Geometry check sheet. Reference: the model listing, model coordinates, mm. Give positions to 0.01 mm unless a question says otherwise; leave off trailing zeros. Order: outer loops, then holes, each group sorted by start corner. A loop starts at its lowest first (then second) coordinate and runs counter-clockwise, first axis right, second up. Notation, with made-up numbers: M 6.5,17 L 16.5,17 A26 ccw 16.5,42 Z; hole C -5,10 d2. An arc over 180 degrees is marked long. Answer as CSV lines item,"result". Start each with the question number.
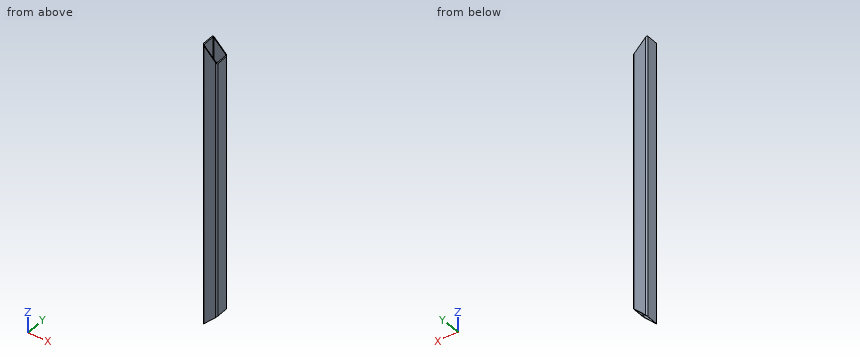
Autodesk Inventor part; units mm, degrees
ref_plane "Piano iniziale" through (0, 0, 0) normal (0, 0, 1) x (1, 0, 0)
ref_plane "Piano finale" through (0, 0, 800) normal (0, 0, 1) x (1, 0, 0)
ref_plane "YZ Plane" through (0, 0, 0) normal (1, 0, 0) x (0, 1, 0)
ref_plane "Piano iniziale" through (0, 0, 0) normal (0, 0, 1) x (1, 0, 0)
ref_plane "Piano finale" through (0, 0, 800) normal (0, 0, 1) x (1, 0, 0)
sketch "Schizzo" plane through (0, 0, 0) normal (0, 0, 1) x (1, 0, 0)
  line L0 (-20, -16) -> (-20, 16)
  line L1 (-16, 20) -> (16, 20)
  line L2 (20, 16) -> (20, -16)
  line L3 (16, -20) -> (-16, -20)
  arc A0 (-20, -16) -> (-16, -20) centre (-16, -16) ccw
  arc A1 (20, 16) -> (16, 20) centre (16, 16) ccw
  arc A2 (-16, 20) -> (-20, 16) centre (-16, 16) ccw
  arc A3 (16, -20) -> (20, -16) centre (16, -16) ccw
  arc A4 (-16, 18) -> (-18, 16) centre (-16, 16) ccw
  line L4 (-16, 18) -> (16, 18)
  arc A5 (18, 16) -> (16, 18) centre (16, 16) ccw
  line L5 (18, 16) -> (18, -16)
  arc A6 (16, -18) -> (18, -16) centre (16, -16) ccw
  line L6 (16, -18) -> (-16, -18)
  arc A7 (-18, -16) -> (-16, -18) centre (-16, -16) ccw
  line L7 (-18, -16) -> (-18, 16)
  line L8 (0, 29.1598) -> (0, -29.1598) construction
  line L9 (-29.1598, 0) -> (29.1598, 0) construction
  dimension "d7" = 4
  dimension "d9" = 40
  dimension "d11" = 40
  dimension "d12" = 2
  dimension "d15" = 20
  dimension "d16" = 20
extrude "Corpo" add sketch "Schizzo" along normal up to surface (800 mm away) from surface at 0
sketch "Sketch3" plane through (0, 0, 0) normal (0, 0, 1) x (1, 0, 0)
  line L0 (0, 0) -> (10, 0)
ref_plane "Work Plane3" through (0, 0, 0) normal (0, -1, 0) x (1, 0, 0)
sketch "Sketch4" plane through (0, 0, 0) normal (0, -1, 0) x (1, 0, 0)
  line L0 (-2, 0) -> (12, 0)
  line L1 (-2, 800) -> (12, 800)
  dimension "d18" = 800
sketch "Schizzo5" plane through (-16, -20, 0) normal (0, -1, 0) x (1, 0, 0)
  line L0 (-4, 0) -> (-4, 800)
  line L1 (-4, 0) -> (0, 0)
  line L2 (-4, 800) -> (0, 800)
  line L3 (-4, 800) -> (0, 800)
  line L4 (-4, 800) -> (46.6766, 749.3234)
  line L5 (-4, 800) -> (67.6675, 800) construction
  line L6 (46.6766, 749.3234) -> (46.6766, 833.8871)
  line L7 (46.6766, 833.8871) -> (-4, 800)
  line L8 (-4, 0) -> (55.8193, 59.8193)
  line L9 (-4, 0) -> (80.5973, 0) construction
  line L10 (55.8193, 59.8193) -> (55.8193, -51.0015)
  line L11 (55.8193, -51.0015) -> (-4, 0)
  point P0 (16, 0)
  dimension "d19" = 45
  dimension "d20" = 45
extrude "Estrusione2" cut sketch "Schizzo5" against normal up to next
equation "\"d7\" = G_IR"
equation "\"d9\" = G_W"
equation "\"d11\" = G_H"
equation "\"d12\" = G_T"
equation "\"d15\" = 0.5 * d9"
equation "\"d16\" = 0.5 * d11"
equation "\"d3\" = G_L"
equation "\"G_W\" = 40"
equation "\"G_H\" = 40"
equation "\"G_T\" = 2"
equation "\"G_IR\" = 4"
equation "\"G_L\" = d18"
equation "\"G_OFFSET_START\" = 0"
equation "\"G_OFFSET_END\" = 0"
properties part number "ISO 10799-2 - 40x40x2 - 800" material "Acciaio, Dolce"
Item 1: Section check B-B on z = 219.5. Record the boundary of the cut face in (x, y), then the cut area to 3 significant figures.
Item 2: Scan lines: line 1 along Y through (x, z) = (8, 313.5); line 2 along Y through (x, z) = (17, 94.5). Record each from-to range of solid material in increasing order.
Item 3: Section check A-A on x = -10. Record the boundary of the cut face in (y, z), then the cut area to 3 significant figures.
Item 4: Section check C-C on y = -1. Record the boundary of the cut face in (x, z), then the cut area to 3 significant figures.
Numbers:
1,outline,"M -20,-16 A4 ccw -16,-20 L 16,-20 A4 ccw 20,-16 L 20,16 A4 ccw 16,20 L -16,20 A4 ccw -20,16 Z; hole M -18,-16 A2 ccw -16,-18 L 16,-18 A2 ccw 18,-16 L 18,16 A2 ccw 16,18 L -16,18 A2 ccw -18,16 Z"
1,area,"294 mm2"
2,line 1,"-20 to -18, 18 to 20"
2,line 2,"-19.87 to -17.73, 17.73 to 19.87"
3,outline,"M -20,10 L -18,10 L -18,790 L -20,790 Z; M 18,10 L 20,10 L 20,790 L 18,790 Z"
3,area,"3,120 mm2"
4,outline,"M -20,0 L -18,2 L -18,798 L -20,800 Z; M 18,38 L 20,40 L 20,760 L 18,762 Z"
4,area,"3,040 mm2"
